Can you work these out from the model? Positions are in its coordinate system, mm. A direction names the side the tool comes from. Coordinates: 2 decimals unless noted, no trailing zeros. Write each loop counter-clockwise with the first axis right and the second up, starting at its lowest first coordinate (ties: lowest second). Pieces come first, ordered by that corner, then holes. Notation, with made-up numbers: (-35.5, -4.75) -> (-25.5, -4.75) arc R22 ccw to (-25.5, 30.25) -> close; hole circle Ø3 at (60, 58). An arc over 180 degrees is marked (long way). Use one line per item in the form item = value.
Autodesk Inventor part; units mm, degrees
ref_plane "YZ Plane" through (0, 0, 0) normal (1, 0, 0) x (0, 1, 0)
ref_plane "XZ Plane" through (0, 0, 0) normal (0, 1, 0) x (-1, 0, 0)
ref_plane "XY Plane" through (0, 0, 0) normal (0, 0, 1) x (1, 0, 0)
sketch "Esquisse1" plane through (0, 0, 0) normal (0, 0, 1) x (1, 0, 0)
  line L0 (0, -47.8) -> (0, 118.8)
  line L1 (-27.8, 0) -> (145.8, 0)
  line L2 (0, 92) -> (105, 92)
  line L3 (105, 92) -> (105, 0)
  line L4 (105, 0) -> (0, 0)
  line L5 (0, 0) -> (0, 92)
  line L6 (56.1007, 59.272) -> (61.1007, 59.272)
  line L7 (61.1007, 59.272) -> (61.1007, 8.472)
  line L8 (61.1007, 8.472) -> (56.1007, 8.472)
  line L9 (56.1007, 8.472) -> (56.1007, 59.272)
  line L10 (0, 92) -> (118, 92)
  line L11 (118, 92) -> (118, -21)
  line L12 (118, -21) -> (0, -21)
  line L13 (0, -21) -> (0, 92)
  line L14 (54.1007, 60.572) -> (63.1007, 60.572)
  line L15 (63.1007, 60.572) -> (63.1007, 7.172)
  line L16 (63.1007, 7.172) -> (54.1007, 7.172)
  line L17 (54.1007, 7.172) -> (54.1007, 60.572)
  line L18 (-3, 95) -> (121, 95)
  line L19 (121, 95) -> (121, -24)
  line L20 (121, -24) -> (-3, -24)
  line L21 (-3, -24) -> (-3, 95)
  line L22 (0, 92) -> (118, 92)
  line L23 (118, 92) -> (118, -21)
  line L24 (118, -21) -> (0, -21)
  line L25 (0, -21) -> (0, 92)
  line L26 (57.2447, 8.472) -> (59.9567, 8.472)
  line L27 (59.9567, 59.272) -> (57.2447, 59.272)
  line L28 (56.1007, 33.3434) -> (56.1007, 31.8605)
  line L29 (61.1007, 31.8605) -> (61.1007, 33.3434)
  circle A0 centre (58.6009, 4.8718) radius 1.3752
  circle A1 centre (58.601, 62.8718) radius 1.3753
  circle A2 centre (9.6007, 62.872) radius 1.375
  circle A3 centre (9.6008, 4.8721) radius 1.3752
  circle A4 centre (9.6008, 4.8721) radius 1.8752
  circle A5 centre (9.6007, 62.872) radius 1.875
  circle A6 centre (58.601, 62.8718) radius 1.8753
  circle A7 centre (58.6009, 4.8718) radius 1.8752
  point P0 (0, 0)
  point P1 (58.6007, 59.272)
  dimension "d0" = 92
  dimension "d1" = 105
  dimension "d6" = 13
  dimension "d7" = 21
  dimension "d8" = 2
  dimension "d9" = 1.3
  dimension "d11" = 1.3
  dimension "d12" = 3
  dimension "d13" = 3
  dimension "d14" = 3
  dimension "d15" = 3
  dimension "d77" = 2
  dimension "d78" = 0.5
  dimension "d79" = 0.5
  dimension "d80" = 0.5
  dimension "d81" = 0.5
extrude "Extrusion1" add sketch "Esquisse1" along normal blind 4 contours L0 L20 L21 L1 | L12 L11 L1 L19 L20 L0 | L0 L1 L11 L12 | L1 L21 L18 L0 | L0 L2 L3 L1 | L0 L18 L19 L1 L11 L10 L2 | L3 L10 L11 L1
sketch "Esquisse2" plane through (0, 0, 4) normal (0, 0, 1) x (1, 0, 0)
  line L0 (-3, -24) -> (121, -24)
  line L1 (-3, 95) -> (121, 95)
  line L2 (121, 95) -> (121, -24)
  line L3 (121, -24) -> (-3, -24)
  line L4 (-3, -24) -> (-3, 95)
  line L5 (0, 92) -> (118, 92)
  line L6 (118, 92) -> (118, -21)
  line L7 (118, -21) -> (0, -21)
  line L8 (0, -21) -> (0, 92)
  point P0 (0, 0)
  dimension "d18" = 3
  dimension "d19" = 3
  dimension "d20" = 3
  dimension "d21" = 3
extrude "Extrusion2" add sketch "Esquisse2" against normal blind 27
sketch "Esquisse4" plane through (-3, -24, 4) normal (0, -1, 0) x (1, 0, 0)
  line L0 (27.38, -19.5) -> (27.38, -6) construction
  line L1 (27.38, -6) -> (11.5, -6) construction
  line L2 (11.5, -6) -> (11.5, -19.5) construction
  line L3 (62.1007, -19.5) -> (12.1007, -19.5) construction
  line L4 (9.1005, -19.5) -> (15.101, -19.5) construction
  line L5 (41.19, -4.01) -> (35.19, -4.01) construction
  line L6 (44.5455, -4.11) -> (31.8345, -4.11) construction
  line L7 (41.19, -2.5351) -> (41.19, -5.6849) construction
  line L8 (35.19, -5.6849) -> (35.19, -2.5351) construction
  circle A0 centre (31.94, -4.51) radius 0.4 construction
  line L9 (31.54, -4.4044) -> (31.54, -9.4204) construction
  line L10 (31.3, -5.5007) -> (31.3, -19.2199) construction
  line L11 (31.3, -5.3465) -> (31.3, -5.5636) construction
  line L12 (31.7209, -4.66) -> (31.5122, -4.66) construction
  line L13 (31.7172, -4.66) -> (31.5053, -4.66) construction
  line L14 (30.64, -9.7204) -> (30.64, -12.7204) construction
  line L15 (30.64, -12.7204) -> (31.3599, -12.7204) construction
  line L16 (31.322, -9.7204) -> (30.64, -9.7204) construction
  line L17 (44.44, -9.27) -> (44.44, -14.39) construction
  line L18 (63.74, -12.7204) -> (63.74, -9.7204) construction
  line L19 (63.08, -19.182) -> (63.08, -5.5251) construction
  line L20 (60.2447, -19.5) -> (62.9567, -19.5) construction
  line L21 (63.08, -18.9857) -> (63.08, -19.517) construction
  line L22 (59.1017, -19.5) -> (65.1003, -19.5) construction
  line L23 (63.08, -4.6635) -> (63.08, -6.647) construction
  circle A1 centre (62.4398, -4.5101) radius 0.4002 construction
  line L24 (62.84, -9.4204) -> (62.84, -4.4044) construction
  line L25 (62.8795, -4.66) -> (62.5088, -4.66) construction
  line L26 (63.08, -4.6726) -> (63.08, -4.66) construction
  line L27 (62.5455, -4.11) -> (49.8345, -4.11) construction
  circle A2 centre (49.94, -4.51) radius 0.4 construction
  line L28 (49.54, -4.4044) -> (49.54, -9.4204) construction
  line L29 (64.08, -20) -> (48.54, -20)
  line L30 (48.54, -20) -> (48.54, -3.61)
  line L31 (48.54, -3.61) -> (64.08, -3.61)
  line L32 (64.08, -3.61) -> (64.08, -20)
  line L33 (45.88, -20) -> (30.3, -20)
  line L34 (30.3, -20) -> (30.3, -3.61)
  line L35 (30.3, -3.61) -> (45.88, -3.61)
  line L36 (45.88, -3.61) -> (45.88, -20)
  line L37 (44.88, -5.5659) -> (44.88, -19.1471)
  line L38 (27.88, -20) -> (11, -20) construction
  line L39 (11, -20) -> (11, -5.5) construction
  line L40 (11, -5.5) -> (27.88, -5.5) construction
  line L41 (27.88, -5.5) -> (27.88, -20) construction
  line L42 (27.88, -20) -> (11, -20)
  line L43 (11, -20) -> (11, -5.5)
  line L44 (11, -5.5) -> (27.88, -5.5)
  line L45 (27.88, -5.5) -> (27.88, -20)
  point P0 (3, -4)
  dimension "d52" = 0.5
  dimension "d53" = 1
  dimension "d54" = 0.5
  dimension "d55" = 1
  dimension "d56" = 1
  dimension "d57" = 1
  dimension "d59" = 0.5
  dimension "d60" = 0.5
  dimension "d61" = 0.5
  dimension "d62" = 0.5
  dimension "d63" = 0.5
  dimension "d64" = 0.5
extrude "Extrusion4" cut sketch "Esquisse4" against normal blind 27
sketch "Esquisse5" plane through (-3, -24, 4) normal (-1, 0, 0) x (0, 0, 1)
  line L0 (-13.62, 51.6049) -> (-13.62, 65.2689)
  line L1 (-19.17, 63.3546) -> (-19.17, 58.0099)
  line L2 (-19.17, 57.98) -> (-19.17, 53.5054)
  line L3 (-16.9746, 76.7653) -> (-16.9746, 82.8881)
  line L4 (-19.7386, 82.3643) -> (-19.7386, 79.9819)
  line L5 (-19.7386, 79.6728) -> (-19.7386, 77.3076)
  line L6 (-17.0251, 50.93) -> (-14.2949, 50.93)
  line L7 (-14.2811, 65.93) -> (-17.0251, 65.93)
  line L8 (-18.2776, 75.8396) -> (-17.9619, 75.8396)
  line L9 (-17.9553, 83.8204) -> (-18.271, 83.8204)
  line L10 (-22.395, 47.43) -> (-10.395, 47.43)
  line L11 (-10.395, 47.43) -> (-10.395, 69.43)
  line L12 (-10.395, 69.43) -> (-22.395, 69.43)
  line L13 (-22.395, 69.43) -> (-22.395, 47.43)
  line L14 (-22.3566, 72.8396) -> (-14.3566, 72.8396)
  line L15 (-14.3566, 72.8396) -> (-14.3566, 86.8396)
  line L16 (-14.3566, 86.8396) -> (-22.3566, 86.8396)
  line L17 (-22.3566, 86.8396) -> (-22.3566, 72.8396)
  point P0 (-4, 24)
  point P1 (-16.395, 69.43)
  point P2 (-18.1197, 75.8396)
  dimension "d67" = 22
  dimension "d68" = 12
  dimension "d69" = 3.225
  dimension "d70" = 3.5
  dimension "d71" = 14
  dimension "d72" = 8
  dimension "d73" = 2.618
  dimension "d74" = 3
extrude "Extrusion5" cut sketch "Esquisse5" against normal blind 27
sketch "Esquisse6" plane through (-3, 95, 4) normal (0, 1, 0) x (1, 0, 0)
  line L0 (121, 4) -> (121, 27)
  line L1 (121, 27) -> (121, 0)
  line L2 (124, 0) -> (0, 0)
  line L3 (3, 4) -> (121, 4)
  line L4 (121, 4) -> (71, 4)
  line L5 (71, 4) -> (71, 21)
  line L6 (71, 21) -> (121, 21)
  line L7 (121, 21) -> (121, 4)
  line L8 (71, 21) -> (88, 21)
  line L9 (88, 21) -> (88, 15)
  line L10 (88, 15) -> (71, 15)
  line L11 (71, 15) -> (71, 21)
  line L12 (121, 21) -> (99, 21)
  line L13 (99, 21) -> (99, 13)
  line L14 (99, 13) -> (121, 13)
  line L15 (121, 13) -> (121, 21)
  point P0 (71, 12.5)
  point P1 (99, 21)
  point P2 (88, 21)
  dimension "d82" = 50
  dimension "d83" = 17
  dimension "d84" = 8
  dimension "d85" = 22
  dimension "d86" = 17
  dimension "d87" = 6
extrude "Extrusion6" cut sketch "Esquisse6" against normal blind 3 contours L14 L13 L6 L0 | L5 L6 L9 L10
sketch "Esquisse7" plane through (121, -24, 4) normal (1, 0, 0) x (0, 0, -1)
  line L0 (22, 74) -> (13, 74)
  line L1 (13, 59) -> (22, 59)
  line L2 (22, 59) -> (22, 74)
  line L3 (0, 119) -> (27, 119)
  line L4 (13, 74) -> (13, 59)
  line L5 (0, 0) -> (0, 119)
  point P0 (4, 24)
  point P1 (13, 66.5)
  dimension "d90" = 60
  dimension "d91" = 45
  dimension "d92" = 13
  dimension "d93" = 9
extrude "Extrusion7" cut sketch "Esquisse7" against normal blind 3
sketch "Esquisse8" plane through (0, 0, -23) normal (0, 0, -1) x (-1, 0, 0)
  line L0 (-1.5, 90.5) -> (1.5, 90.5)
  line L1 (1.5, 90.5) -> (1.5, 93.5)
  line L2 (1.5, 93.5) -> (-1.5, 93.5)
  line L3 (-1.5, 93.5) -> (-1.5, 90.5)
  line L4 (-118, 92) -> (0, 92)
  line L5 (-1.5, 90.5) -> (1.5, 93.5) construction
  line L6 (1.5, 90.5) -> (-1.5, 93.5) construction
  line L7 (-1.5, -19.5) -> (1.5, -19.5)
  line L8 (1.5, -19.5) -> (1.5, -22.5)
  line L9 (1.5, -22.5) -> (-1.5, -22.5)
  line L10 (-1.5, -22.5) -> (-1.5, -19.5)
  line L11 (-1.5, -19.5) -> (1.5, -22.5) construction
  line L12 (1.5, -19.5) -> (-1.5, -22.5) construction
  line L13 (-116.5, 93.5) -> (-119.5, 93.5)
  line L14 (-119.5, 93.5) -> (-119.5, 90.5)
  line L15 (-119.5, 90.5) -> (-116.5, 90.5)
  line L16 (-116.5, 90.5) -> (-116.5, 93.5)
  line L17 (-118, -21) -> (-118, 92)
  line L18 (-116.5, 93.5) -> (-119.5, 90.5) construction
  line L19 (-119.5, 93.5) -> (-116.5, 90.5) construction
  line L20 (-119.5, -19.5) -> (-116.5, -19.5)
  line L21 (-116.5, -19.5) -> (-116.5, -22.5)
  line L22 (-116.5, -22.5) -> (-119.5, -22.5)
  line L23 (-119.5, -22.5) -> (-119.5, -19.5)
  line L24 (-119.5, -19.5) -> (-116.5, -22.5) construction
  line L25 (-116.5, -19.5) -> (-119.5, -22.5) construction
  line L26 (1.5, 93.5) -> (-13.5, 93.5)
  line L27 (-13.5, 93.5) -> (-13.5, 78.5)
  line L28 (-13.5, 78.5) -> (1.5, 78.5)
  line L29 (1.5, 78.5) -> (1.5, 93.5)
  line L30 (1.5, -22.5) -> (-13.5, -22.5)
  line L31 (-13.5, -22.5) -> (-13.5, -7.5)
  line L32 (-13.5, -7.5) -> (1.5, -7.5)
  line L33 (1.5, -7.5) -> (1.5, -22.5)
  line L34 (-119.5, -22.5) -> (-104.5, -22.5)
  line L35 (-104.5, -22.5) -> (-104.5, -7.5)
  line L36 (-104.5, -7.5) -> (-119.5, -7.5)
  line L37 (-119.5, -7.5) -> (-119.5, -22.5)
  line L38 (-119.5, 93.5) -> (-104.5, 93.5)
  line L39 (-104.5, 93.5) -> (-104.5, 78.5)
  line L40 (-104.5, 78.5) -> (-119.5, 78.5)
  line L41 (-119.5, 78.5) -> (-119.5, 93.5)
  point P0 (0, 0)
  point P1 (0, -21)
  point P2 (-118, 78.5)
  point P3 (-104.5, 92)
  point P4 (-116.5, 92)
  point P5 (-118, 90.5)
  point P6 (-118, -7.5)
  point P7 (-118, -19.5)
  point P8 (1.5, 90.5)
  point P9 (-1.5, 92)
  point P10 (-13.5, 92)
  point P11 (-1.5, 93.5)
  dimension "d96" = 3
  dimension "d97" = 3
  dimension "d98" = 3
  dimension "d99" = 3
  dimension "d100" = 3
  dimension "d101" = 3
  dimension "d102" = 3
  dimension "d105" = 15
  dimension "d106" = 15
  dimension "d107" = 15
  dimension "d108" = 15
  dimension "d109" = 15
extrude "Extrusion8" cut sketch "Esquisse8" against normal blind 5
sketch "Esquisse10" plane through (0, 0, 0) normal (0, 0, -1) x (-1, 0, 0)
  line L0 (0, -21) -> (0, -7.5)
  line L1 (0, -21) -> (-4, -21)
  line L2 (-4, -21) -> (-4, -17)
  line L3 (-4, -17) -> (0, -17)
  line L4 (0, -17) -> (0, -21)
  line L5 (-118, -21) -> (-61.08, -21)
  line L6 (-118, -21) -> (-114, -21)
  line L7 (-114, -21) -> (-114, -17)
  line L8 (-114, -17) -> (-118, -17)
  line L9 (-118, -17) -> (-118, -21)
  line L10 (0, -21) -> (0, 92)
  line L11 (0, 92) -> (-4, 92)
  line L12 (-4, 92) -> (-4, 88)
  line L13 (-4, 88) -> (0, 88)
  line L14 (0, 88) -> (0, 92)
  line L15 (-118, 92) -> (-118, -21)
  line L16 (-118, 92) -> (-114, 92)
  line L17 (-114, 92) -> (-114, 88)
  line L18 (-114, 88) -> (-118, 88)
  line L19 (-118, 88) -> (-118, 92)
  line L20 (0, -21) -> (-118, -21)
  line L21 (-118, -21) -> (-118, 92)
  line L22 (-118, 92) -> (0, 92)
  line L23 (0, 92) -> (0, -21)
  point P0 (0, 0)
  point P1 (0, -17)
  dimension "d119" = 4
  dimension "d120" = 4
  dimension "d121" = 4
  dimension "d122" = 4
  dimension "d123" = 4
  dimension "d124" = 4
  dimension "d125" = 4
  dimension "d126" = 4
extrude "Extrusion10" cut sketch "Esquisse10" against normal blind 1 contours L3 L2 L20 L5 L7 L8 L15 L18 L17 L22 L12 L13 L10 L0
fillet "Congé1" radius 2 4 edges at (-3, -24, -9.5) (121, -24, -9.5) (-3, 95, -9.5) (121, 95, -9.5)
sketch "Esquisse11" plane through (0, 0, 4) normal (0, 0, 1) x (1, 0, 0)
  line L0 (106, 80) -> (116, 80)
  line L1 (116, 80) -> (116, 90)
  line L2 (116, 90) -> (106, 90)
  line L3 (106, 90) -> (106, 80)
  line L4 (119, 95) -> (-1, 95)
  line L5 (121, -22) -> (121, 93)
  line L6 (116, -19) -> (106, -19)
  line L7 (106, -19) -> (106, -9)
  line L8 (106, -9) -> (116, -9)
  line L9 (116, -9) -> (116, -19)
  line L10 (-1, -24) -> (119, -24)
  line L11 (12, -9) -> (2, -9)
  line L12 (2, -9) -> (2, -19)
  line L13 (2, -19) -> (12, -19)
  line L14 (12, -19) -> (12, -9)
  line L15 (-3, 93) -> (-3, -22)
  line L16 (12, 90) -> (2, 90)
  line L17 (2, 90) -> (2, 80)
  line L18 (2, 80) -> (12, 80)
  line L19 (12, 80) -> (12, 90)
  point P0 (0, 0)
  point P1 (111, 90)
  point P2 (111, -19)
  dimension "d130" = 10
  dimension "d131" = 10
  dimension "d132" = 5
  dimension "d133" = 5
  dimension "d134" = 10
  dimension "d135" = 10
  dimension "d136" = 5
  dimension "d137" = 5
  dimension "d138" = 10
  dimension "d139" = 10
  dimension "d140" = 5
  dimension "d141" = 5
  dimension "d142" = 5
  dimension "d143" = 10
  dimension "d144" = 10
  dimension "d145" = 5
extrude "Extrusion11" cut sketch "Esquisse11" against normal blind 2
properties part number "coque_RPI"
Q1. Thinking about a two-plate mould opening in X: for faces 1 (the flat face through (27.3, -23, -8)), 2 (the flat face through (-2, 56, -18.357)), which applies, released by +X, released by -X, zero draft, split by the parting line, or undercut?
Return value:
face_1 = undercut
face_2 = zero draft
Q2. Suppose I cut it at D-D (y = 15.5). Write out the boundary of the cut face in (x, z), then the cut area to 3 significant figures.
Return value:
outline = (-3, -23) -> (0, -23) -> (0, 1) -> (54.1, 1) -> (54.1, 4) -> (-3, 4) -> close; (63.1, 1) -> (118, 1) -> (118, -23) -> (121, -23) -> (121, 4) -> (63.1, 4) -> close
area = 489 mm2
Q3. Suppose I cut it at A-A (y = 41). Write out the boundary of the cut face in (x, z) (3 decimals), then the cut area to 3 significant figures.
Return value:
outline = (-3, -23) -> (0, -23) -> (0, -18.395) -> (-3, -18.395) -> close; (-3, -6.395) -> (0, -6.395) -> (0, 1) -> (54.101, 1) -> (54.101, 4) -> (-3, 4) -> close; (63.101, 1) -> (118, 1) -> (118, -9) -> (121, -9) -> (121, 4) -> (63.101, 4) -> close; (118, -23) -> (121, -23) -> (121, -18) -> (118, -18) -> close
area = 426 mm2
Q4. Will these pins go through, and if not, where does the flat tip stop? pin 1 (1.2 mm diameter, centred on x = 1, y = 91, fed in from -Z); pin 2 (10 mm diameter, centred on x = 15, z = -9.5, fed in from -Y); pin 3 (4 mm diameter, centred on y = 61, z = -15.5, fed in from -X); pin 4 (1.5 mm diameter, centred on x = 120, z = -15.5, fed in from -Y).
Return value:
pin_1 = 0
pin_2 = 92
pin_3 = -3
pin_4 = -23.98
Q5. Suppose I cut it at C-C (x = 39). Write out the boundary of the cut face in (y, z).
Return value:
outline = (-24, -23) -> (-21, -23) -> (-21, -16) -> (-24, -16) -> close; (-24, 0.39) -> (-21, 0.39) -> (-21, 1) -> (92, 1) -> (92, -23) -> (95, -23) -> (95, 4) -> (-24, 4) -> close
Q6. If I drill on line 1 (Y direction, x = 94, z = -14.5); line 2 (Y direction, x = 9, z = -21.25); line 3 (X direction, y = 30, z = -4), over which ranges is the centre line in solid material (lowest first)? Write a range as from..to.
Return value:
line_1 = -24..-21, 92..95
line_2 = -24..-22.5, 93.5..95
line_3 = -3..0, 118..121
Q7. Suppose I cut it at B-B (z = -5). Write out the boundary of the cut face in (x, y).
Return value:
outline = (-3, -22) arc R2 ccw to (-1, -24) -> (8, -24) -> (8, -21) -> (0, -21) -> (0, 92) -> (118, 92) -> (118, -21) -> (61.08, -21) -> (61.08, -24) -> (119, -24) arc R2 ccw to (121, -22) -> (121, 93) arc R2 ccw to (119, 95) -> (-1, 95) arc R2 ccw to (-3, 93) -> close; (24.88, -24) -> (27.3, -24) -> (27.3, -21) -> (24.88, -21) -> close; (42.88, -24) -> (45.54, -24) -> (45.54, -21) -> (42.88, -21) -> close
Q8. For faces 3 (the flat face through (85, 94, -14)), 4 (the flat face through (2, -19, 0)), 5 (the flat face through (59, 60.572, 2)), 6 (the flat face through (42.88, -23, -8)), which set-ups out of +Z, -Z, +X, -X, +Y, -Y let a thin tool reach every point of the face, with its end or its side?
Return value:
face_3 = +Y
face_4 = -Z
face_5 = +Z, -Z
face_6 = -Y
